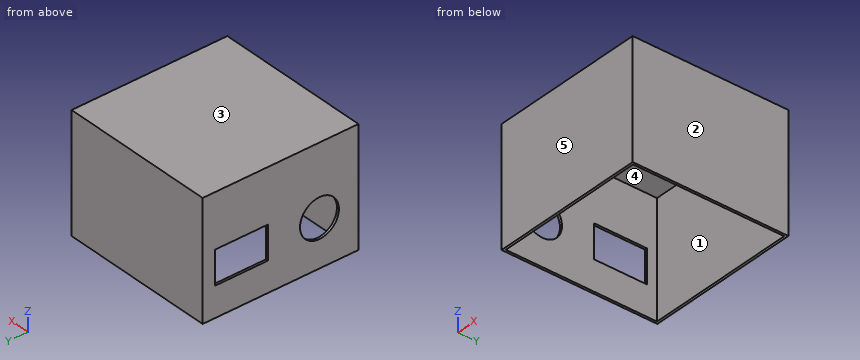
Autodesk Inventor part; units mm, degrees
sketch "Sketch2" plane through (0, 0, 0) normal (0, 0, 1) x (1, 0, 0)
  line L0 (100, -100) -> (-100, -100)
  line L1 (-100, -100) -> (-100, 100)
  line L2 (-100, 100) -> (100, 100)
  line L3 (100, 100) -> (100, -100)
  line L4 (100, -100) -> (-100, 100) construction
  line L5 (-100, -100) -> (100, 100) construction
  point P0 (0, 0)
  dimension "d0" = 200
  dimension "d1" = 200
extrude "Extrusion1" add sketch "Sketch2" along normal blind 150
sketch "Sketch3" plane through (0, 0, 0) normal (0, 0, -1) x (-1, 0, 0)
  line L0 (-97, 97) -> (97, 97)
  line L1 (97, 97) -> (97, -97)
  line L2 (97, -97) -> (-97, -97)
  line L3 (-97, -97) -> (-97, 97)
  line L4 (-97, 97) -> (97, -97) construction
  line L5 (97, 97) -> (-97, -97) construction
  line L6 (-100, 100) -> (100, 100) construction
  line L7 (-100, -100) -> (-100, 100) construction
  line L8 (100, -100) -> (-100, -100) construction
  line L9 (100, 100) -> (100, -100) construction
  point P0 (0, 0)
  dimension "d4" = 3
  dimension "d5" = 3
extrude "Extrusion2" cut sketch "Sketch3" against normal blind 147
sketch "Sketch4" plane through (-100, -100, 0) normal (-1, 0, 0) x (0, 0, 1)
  line L0 (0, 200) -> (0, 0) construction
  line L1 (0, 0) -> (150, 0) construction
  line L2 (150, 200) -> (150, 0) construction
  line L3 (0, 200) -> (150, 200) construction
  line L4 (38.5, 116) -> (81.5, 116)
  line L5 (81.5, 116) -> (81.5, 184)
  line L6 (81.5, 184) -> (38.5, 184)
  line L7 (38.5, 184) -> (38.5, 116)
  line L8 (38.5, 116) -> (81.5, 184) construction
  line L9 (81.5, 116) -> (38.5, 184) construction
  circle A0 centre (60, 50) radius 25
  line L10 (0, 200) -> (0, 0) construction
  point P0 (0, 100)
  point P1 (60, 150)
  dimension "d8" = 43
  dimension "d9" = 68
  dimension "d10" = 50
  dimension "d11" = 60
  dimension "d12" = 60
  dimension "d13" = 200
  dimension "d14" = 50
  dimension "d15" = 50
extrude "Extrusion3" cut sketch "Sketch4" against normal up to surface (3 mm away)
sketch "Sketch5" plane through (-100, -100, 0) normal (0, -1, 0) x (1, 0, 0)
  point P0 (100, 0)
sketch "Sketch6" plane through (0, 0, 0) normal (0, 0, -1) x (-1, 0, 0)
  line L0 (97, 97) -> (97, -97) construction
  line L1 (97, -97) -> (-97, -97) construction
  line L2 (-97, -97) -> (-97, 97) construction
  line L3 (-97, 97) -> (97, 97) construction
  line L4 (-100, 100) -> (100, 100) construction
  line L5 (-100, -100) -> (-100, 100) construction
  line L6 (100, -100) -> (-100, -100) construction
  line L7 (100, 100) -> (100, -100) construction
  point P0 (0, 0)
equation "\"d15\" = 0.25 * d13"
properties part number "P022_Coque_boitier"
Could you check a few things on this model? Use its own coordinates, in mm. Face numbers are marked on the shaded views. A direction names the side the tool comes from. Coordinates: 2 decimals unless noted, no trailing zeros. Loops run counter-clockwise (first coordinate to the right, second up) from the corner with the lowest first, then second, coordinate; pieces in that order, holes last.
1. For the marked faces 1 and 2, which set-ups out of +Z, -Z, +X, -X, +Y, -Y let a thin tool reach every point of the face, with its end or its side?
2. Imagine slicing it at C-C (x = -80). Please give me the cut outline in (y, z), and give its area (3 significant figures).
3. Imagine slicing it at B-B (y = 20). Please give me the cut outline in (x, z).
4. For P1, Ø5, axis at x = -71.5, y = 78, coming from the -Z side, with a flat end and sliding along its axis, tell me the tip position at first contact or that it passes through.
5. Imagine slicing it at A-A (z = 60). Please give me the cut outline in (x, y), and give its area (3 significant figures).
6. We'd pull the mould along Y, two halves only. Please class the marked faces 3, 4 and 5: released by +Y, released by -Y, zero draft, split by the parting line, or undercut.
7. I need wall thicknesses on L1, parallel to Y at x = -97.85, z = 60; L2, parallel to X at y = 88, z = 88. Which ranges of each line are inside material? Lowest first, please.
Computed values:
1. face 1: -Z
1. face 2: +Z, -Z, +X, +Y, -Y
2. outline: (-100, 0) - (-97, 0) - (-97, 147) - (97, 147) - (97, 0) - (100, 0) - (100, 150) - (-100, 150) - close
2. area: 1,480 mm2
3. outline: (-100, 0) - (-97, 0) - (-97, 38.5) - (-100, 38.5) - close; (-100, 81.5) - (-97, 81.5) - (-97, 147) - (97, 147) - (97, 0) - (100, 0) - (100, 150) - (-100, 150) - close
4. P1: stops at z = 147
5. outline: (-100, -100) - (100, -100) - (100, 100) - (-100, 100) - (-100, 84) - (-97, 84) - (-97, 97) - (97, 97) - (97, -97) - (-97, -97) - (-97, -75) - (-100, -75) - close; (-100, -25) - (-97, -25) - (-97, 16) - (-100, 16) - close
5. area: 2,010 mm2
6. face 3: zero draft
6. face 4: undercut
6. face 5: released by -Y
7. L1: y = -100 to -75, -25 to 16, 84 to 100
7. L2: x = -100 to -97, 97 to 100
